Work out the finished part from the listing and answer in its coordinate system (mm). A direction names the side the tool comes from. Give positions to 0.01 mm unless a question says otherwise; leave off trailing zeros. Order: outer loops, then holes, each group sorted by start corner. A loop starts at its lowest first (then second) coordinate and runs counter-clockwise, first axis right, second up. Notation, with made-up numbers: (40, 78) - (46, 78) arc R17 cw to (46, 105) - close; hole circle Ø4 at (34, -28.5). An arc over 180 degrees is marked (long way). Put each result on its own line as item: value.
Autodesk Inventor part; units mm, degrees
ref_plane "YZ Plane" through (0, 0, 0) normal (1, 0, 0) x (0, 1, 0)
ref_plane "XZ Plane" through (0, 0, 0) normal (0, 1, 0) x (-1, 0, 0)
ref_plane "XY Plane" through (0, 0, 0) normal (0, 0, 1) x (1, 0, 0)
sketch "Sketch1" plane through (0, 0, 0) normal (0, 0, 1) x (1, 0, 0)
  line L0 (-49.7, 49.7) -> (49.7, 49.7)
  line L1 (49.7, 49.7) -> (49.7, -49.7)
  line L2 (49.7, -49.7) -> (-49.7, -49.7)
  line L3 (-49.7, -49.7) -> (-49.7, 49.7)
  line L4 (-49.7, 49.7) -> (49.7, -49.7) construction
  line L5 (49.7, 49.7) -> (-49.7, -49.7) construction
  line L6 (44, -44) -> (-44, -44)
  line L7 (-44, -44) -> (-44, 44)
  line L8 (-44, 44) -> (44, 44)
  line L9 (44, 44) -> (44, -44)
  line L10 (44, -44) -> (-44, 44) construction
  line L11 (-44, -44) -> (44, 44) construction
  circle A0 centre (-44, 44) radius 1.75
  circle A1 centre (44, 44) radius 1.75
  circle A2 centre (-44, -44) radius 1.75
  circle A3 centre (44, -44) radius 1.75
  point P0 (0, 0)
  dimension "d0" = 99.4
  dimension "d1" = 99.4
  dimension "d2" = 88
  dimension "d3" = 88
  dimension "d4" = 3.5
  dimension "d5" = 3.5
  dimension "d6" = 3.5
  dimension "d7" = 3.5
extrude "Extrusion1" add sketch "Sketch1" along normal blind 4 contours L0 L1 L2 L3 | A2 L7 L6 | A2 L7 A0 L8 A1 L9 A3 L6 | L6 L7 A2 | A3 L9 L6 | L6 L9 A3 | A0 L8 L7 | L7 L8 A0 | A1 L8 L9 | L9 L8 A1
fillet "Fillet1" radius 4 4 edges at (-49.7, -49.7, 2) (49.7, -49.7, 2) (-49.7, 49.7, 2) (49.7, 49.7, 2)
sketch "Sketch2" plane through (0, 0, 4) normal (0, 0, 1) x (1, 0, 0)
  line L0 (10.125, -10.125) -> (-10.125, -10.125)
  line L1 (-10.125, -10.125) -> (-10.125, 10.125)
  line L2 (-10.125, 10.125) -> (10.125, 10.125)
  line L3 (10.125, 10.125) -> (10.125, -10.125)
  line L4 (10.125, -10.125) -> (-10.125, 10.125) construction
  line L5 (-10.125, -10.125) -> (10.125, 10.125) construction
  line L6 (-15.125, 15.125) -> (15.125, 15.125)
  line L7 (15.125, 15.125) -> (15.125, -15.125)
  line L8 (15.125, -15.125) -> (-15.125, -15.125)
  line L9 (-15.125, -15.125) -> (-15.125, 15.125)
  line L10 (-15.125, 15.125) -> (15.125, -15.125) construction
  line L11 (15.125, 15.125) -> (-15.125, -15.125) construction
  point P0 (0, 0)
  point P1 (0, -15.125)
  dimension "d15" = 20.25
  dimension "d16" = 20.25
  dimension "d17" = 5
extrude "Extrusion2" add sketch "Sketch2" along normal blind 30
fillet "Fillet3" radius 1 4 edges at (-10.125, -10.125, 19) (10.125, -10.125, 19) (10.125, 10.125, 19) (-10.125, 10.125, 19)
fillet "Fillet4" radius 4 8 edges at (15.125, -15.125, 19) (15.125, 15.125, 19) (-15.125, 15.125, 19) (-15.125, -15.125, 19) (0, -15.125, 4) (15.125, 0, 4) (0, 15.125, 4) (-15.125, 0, 4)
sketch "Sketch3" plane through (15.125, -11.125, 34) normal (1, 0, 0) x (0, 0, -1)
  line L0 (30, 22.25) -> (26, 22.25)
  line L1 (0, 0) -> (26, 22.25)
  circle A0 centre (12.4937, 10.6917) radius 2.75
  point P0 (34, 11.125)
  dimension "d22" = 5.5
extrude "Extrusion3" cut sketch "Sketch3" against normal through all
sketch "Sketch4" plane through (-11.125, -15.125, 8) normal (0, -1, 0) x (1, 0, 0)
  line L0 (-4, 26) -> (0, 26)
  line L1 (0, 0) -> (22.25, 0)
  line L2 (0, 26) -> (22.25, 0)
  circle A0 centre (11.125, 13) radius 2.75
  point P0 (11.125, -8)
  point P1 (9.337, 15.0894)
  point P2 (12.913, 10.9106)
  dimension "d25" = 5.5
extrude "Extrusion4" cut sketch "Sketch4" against normal through all
sketch "Sketch5" plane through (0, 0, 4) normal (0, 0, 1) x (1, 0, 0)
  line L0 (-43.5, 24) -> (-33.5, 24)
  line L1 (-33.5, 24) -> (-33.5, 14)
  line L2 (-33.5, 14) -> (-43.5, 14)
  line L3 (-43.5, 14) -> (-43.5, 24)
  line L4 (-48.7, 44.7) -> (-48.7, -44.7)
  line L5 (44.7, 48.7) -> (-44.7, 48.7)
  line L6 (-49.7, 45.7) -> (-49.7, -45.7)
  point P0 (0, 0)
  point P1 (-49.3, 43.8338)
  point P2 (-49.3, -43.8338)
  point P3 (43.8338, 49.3)
  point P4 (-43.8338, 49.3)
  dimension "d31" = 10
  dimension "d32" = 10
  dimension "d33" = 24.7
  dimension "d57" = 6.2
extrude "Extrusion5" cut sketch "Sketch5" against normal blind 10
fillet "Fillet5" radius 2 4 edges at (-43.5, 24, 2) (-33.5, 24, 2) (-33.5, 14, 2) (-43.5, 14, 2)
sketch "Sketch6" plane through (0, 0, 4) normal (0, 0, 1) x (1, 0, 0)
  line L0 (-41.5, 14) -> (-35.5, 14)
  line L1 (-41.5, 14) -> (-49.7, 14)
  line L2 (-49.7, 14) -> (-49.7, 24)
  line L3 (-49.7, 24) -> (-41.5, 24)
  line L4 (-41.5, 24) -> (-41.5, 14)
  line L5 (-49.7, 45.7) -> (-49.7, -45.7)
  point P0 (0, 0)
  point P1 (-35.5, 24)
  point P2 (-49.3, 43.8338)
  point P3 (-49.3, -43.8338)
extrude "Extrusion6" cut sketch "Sketch6" against normal blind 10
sketch "Sketch7" plane through (0, 0, 4) normal (0, 0, 1) x (1, 0, 0)
  arc A0 (11.125, -19.125) -> (19.125, -11.125) centre (11.125, -11.125) ccw
  line L0 (-11.125, -19.125) -> (11.125, -19.125)
  arc A1 (-19.125, -11.125) -> (-11.125, -19.125) centre (-11.125, -11.125) ccw
  line L1 (-19.125, 11.125) -> (-19.125, -11.125)
  arc A2 (-11.125, 19.125) -> (-19.125, 11.125) centre (-11.125, 11.125) ccw
  line L2 (11.125, 19.125) -> (-11.125, 19.125)
  arc A3 (19.125, 11.125) -> (11.125, 19.125) centre (11.125, 11.125) ccw
  line L3 (19.125, -11.125) -> (19.125, 11.125)
  line L4 (-35.5, 14) -> (-49.7, 14)
  line L5 (-49.7, 14) -> (-49.7, -45.7)
  arc A4 (-49.7, -45.7) -> (-45.7, -49.7) centre (-45.7, -45.7) ccw
  line L6 (-45.7, -49.7) -> (45.7, -49.7)
  arc A5 (45.7, -49.7) -> (49.7, -45.7) centre (45.7, -45.7) ccw
  line L7 (49.7, -45.7) -> (49.7, 45.7)
  arc A6 (49.7, 45.7) -> (45.7, 49.7) centre (45.7, 45.7) ccw
  line L8 (45.7, 49.7) -> (-45.7, 49.7)
  arc A7 (-45.7, 49.7) -> (-49.7, 45.7) centre (-45.7, 45.7) ccw
  line L9 (-49.7, 24) -> (-35.5, 24)
  arc A8 (-33.5, 22) -> (-35.5, 24) centre (-35.5, 22) ccw
  line L10 (-33.5, 22) -> (-33.5, 16)
  arc A9 (-35.5, 14) -> (-33.5, 16) centre (-35.5, 16) ccw
  line L11 (-49.7, 12.8) -> (-32.3, 12.8)
  line L12 (-32.3, 12.8) -> (-32.3, 25.2)
  line L13 (-32.3, 25.2) -> (-49.7, 25.2)
  line L14 (-49.7, 25.2) -> (-49.7, 12.8)
  line L15 (-49.7, 45.7) -> (-49.7, 24)
  point P0 (0, 0)
  point P1 (-42.6, 24)
  dimension "d40" = 1.2
  dimension "d41" = 1.2
  dimension "d42" = 1.2
extrude "Extrusion7" add sketch "Sketch7" along normal blind 2 contours A9 L10 A8 L9 L14 L13 L12 L11 L5 L4
fillet "Fillet8" radius 2 2 edges at (-32.3, 25.2, 5) (-32.3, 12.8, 5)
sketch "Sketch8" plane through (0, 0, 4) normal (0, 0, 1) x (1, 0, 0)
  line L0 (45, 6.0205) -> (-45, 6.0205)
  line L1 (-45, 6.0205) -> (-45, -6.0205)
  line L2 (-45, -6.0205) -> (45, -6.0205)
  line L3 (45, -6.0205) -> (45, 6.0205)
  line L4 (45, 6.0205) -> (-45, -6.0205) construction
  line L5 (-45, 6.0205) -> (45, -6.0205) construction
  line L6 (6.0205, -45) -> (-6.0205, -45)
  line L7 (-6.0205, -45) -> (-6.0205, 45)
  line L8 (-6.0205, 45) -> (6.0205, 45)
  line L9 (6.0205, 45) -> (6.0205, -45)
  line L10 (6.0205, -45) -> (-6.0205, 45) construction
  line L11 (-6.0205, -45) -> (6.0205, 45) construction
  point P0 (0, 0)
  dimension "d46" = 90
  dimension "d47" = 12.041
  dimension "d48" = 12.041
  dimension "d49" = 90
hole "Hole1" at (-45, -6.0205, 4) at (45, 6.0205, 4) at (6.0205, -45, 4) at (-6.0205, 45, 4) direction (0, 0, -1) diameter 4.3 end through all countersink diameter 9.4 countersink angle 90
properties part number "Lid"
(1) Determine the mould class of faces 1 (the face through (-16.27, 0.16, 5.2)), 2 (the face through (49.7, 1, 2)), 3 (the face through (-0.358, 12.59, 23.727)) for opening direction Z: pulls with the +Z half, pulls with the -Z half, needs draft (parallel to the pull), parting line crosses it, or undercut.
Geometry check:
face 1: pulls with the +Z half
face 2: needs draft
face 3: undercut
(2) A tool of negligible diameter and unlimited length cuts with its end or side. For faces 4 (the face through (-15.125, 0, 18)), 5 (the face through (13.984, 13.922, 21.182)), 6 (the face through (0, -15.125, 18)), from which of +Z, -Z, +X, -X, +Y, -Y can it reach the whole face along a straight path? Write none if from no direction.
Geometry check:
face 4: +Z, -X, +Y, -Y
face 5: +Z, +X, +Y
face 6: +Z, +X, -X, -Y
(3) Given pin 1 (5 mm diameter, centred on x = -6.02, y = 45, fed in from +Z); pin 2 (3.5 mm diameter, centred on x = 45, y = 6.02, fed in from -Z); pin 3 (5 mm diameter, centred on x = 27, z = 5, fed in from -Y); pin 4 (10 mm diameter, centred on y = 10, z = 20, fed in from +X) (3 decimals), each flat-ended and moving along its own axis, determine where each tip first touches the part or whether it passes through.
Geometry check:
pin 1: stops at z = 1.8
pin 2: passes through
pin 3: stops at y = -49.7
pin 4: stops at x = 15.125
(4) Section B-B, the plane x = 0 is taken. Write down the section's boundary in (y, z) (3 decimals).
Geometry check:
outline: (-49.7, 0) - (49.7, 0) - (49.7, 4) - (19.125, 4) arc R4 cw to (15.125, 8) - (15.125, 18.25) - (10.125, 18.25) - (10.125, 4) - (-10.125, 4) - (-10.125, 18.25) - (-15.125, 18.25) - (-15.125, 8) arc R4 cw to (-19.125, 4) - (-49.7, 4) - close; (-15.125, 23.75) - (-10.125, 23.75) - (-10.125, 34) - (-15.125, 34) - close; (10.125, 23.75) - (15.125, 23.75) - (15.125, 34) - (10.125, 34) - close
(5) Straight lines are drawn through the part: line 1 (Y direction, x = -4, z = 8) (3 decimals); line 2 (X direction, y = 45, z = 1); line 3 (Y direction, x = -45, z = 1). For each, find the intervals that lie inside material, in ascending order.
Geometry check:
line 1: y = -15.125 to -10.125, 10.125 to 15.125
line 2: x = -49.7 to -8.17, -3.87 to 49.7
line 3: y = -49.7 to -8.17, -3.87 to 14, 24 to 49.7
(6) Section A-A, the plane z = 26 is taken. Write down the section's boundary in (x, y) (3 decimals), then the cut area to 3 significant figures.
Geometry check:
outline: (-15.125, -11.125) arc R4 ccw to (-11.125, -15.125) - (11.125, -15.125) arc R4 ccw to (15.125, -11.125) - (15.125, 11.125) arc R4 ccw to (11.125, 15.125) - (-11.125, 15.125) arc R4 ccw to (-15.125, 11.125) - close; hole (-10.125, -9.125) arc R1 ccw to (-9.125, -10.125) - (9.125, -10.125) arc R1 ccw to (10.125, -9.125) - (10.125, 9.125) arc R1 ccw to (9.125, 10.125) - (-9.125, 10.125) arc R1 ccw to (-10.125, 9.125) - close
area: 492 mm²
(7) Section C-C, the plane y = -26 is taken. Write down the section's boundary in (x, z), then the cut area to 3 significant figures.
Geometry check:
outline: (-49.7, 0) - (49.7, 0) - (49.7, 4) - (-49.7, 4) - close
area: 398 mm²
